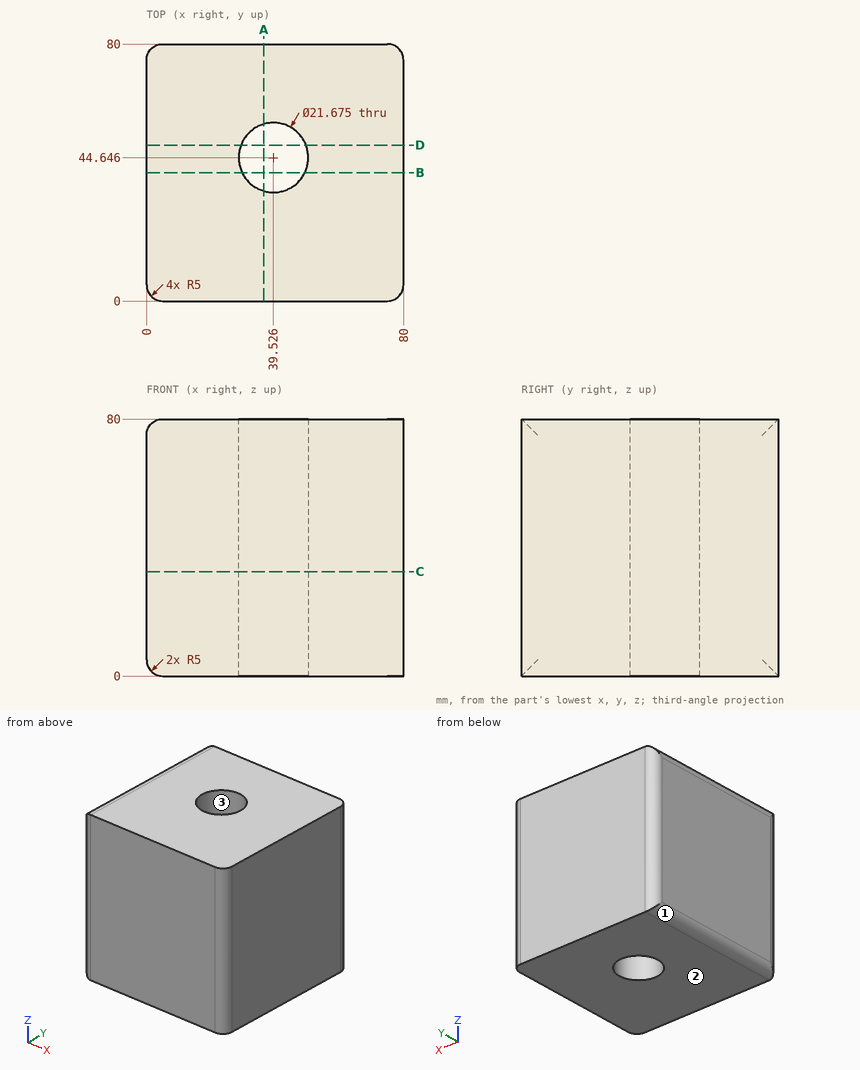
Geometry check sheet. Reference: drawing and pictorial views, mm from the part's lowest x, y, z. Give positions to 0.01 mm unless a question says otherwise; leave off trailing zeros. Loops run counter-clockwise (first coordinate to the right, second up) from the corner with the lowest first, then second, coordinate; pieces in that order, holes last. Notation, with made-up numbers: (26.5, 12.5) - (36.5, 12.5) arc R18 ccw to (36.5, 31.5) - close; hole circle Ø7 at (48, 13). An arc over 180 degrees is marked (long way). Use CSV: the item, a comma, the result in double quotes. Start each with the question number.
Q1. Section check B-B, the plane y = 40. Record the cut outline in (x, z) (1 decimal).
Q2. Section check C-C, the plane z = 32.5. Record the cut outline in (x, y) (1 decimal).
Q3. Scan lines: probe 1 along X at (y, z) = (39, 62) (1 decimal); probe 2 along X at (y, z) = (35.5, 23) (1 decimal); probe 3 along Y at (x, z) = (35, 45). Record each from-to range of solid material in increasing order. Write a range as from..to.
Q4. Section check D-D, the plane y = 48.5. Record the cut outline in (x, z) (1 decimal).
Q5. Release check for a two-part mould opening along X. For the marked faces 1, 2 and 3 record: +X half, -X half, draft (parallel to the pull), parting line (faces both ways), or undercut.
Q6. Section check A-A, the plane x = 36.5. Record the cut outline in (y, z), and give its area (4 significant figures).
Findings below:
1,outline,"(0, 5) arc R5 ccw to (5, 0) - (29.7, 0) - (29.7, 80) - (5, 80) arc R5 ccw to (0, 75) - close; (49.3, 0) - (80, 0) - (80, 80) - (49.3, 80) - close"
2,outline,"(0, 5) arc R5 ccw to (5, 0) - (75, 0) arc R5 ccw to (80, 5) - (80, 75) arc R5 ccw to (75, 80) - (5, 80) arc R5 ccw to (0, 75) - close; hole circle Ø21.7 at (39.5, 44.6)"
3,probe 1,"x = 0..30.3, 48.8..80"
3,probe 2,"x = 0..33.7, 45.3..80"
3,probe 3,"y = 0..34.8, 54.49..80"
4,outline,"(0, 5) arc R5 ccw to (5, 0) - (29.4, 0) - (29.4, 80) - (5, 80) arc R5 ccw to (0, 75) - close; (49.7, 0) - (80, 0) - (80, 80) - (49.7, 80) - close"
5,face 1,"-X half"
5,face 2,"draft"
5,face 3,"undercut"
6,outline,"(0, 0) - (34.24, 0) - (34.24, 80) - (0, 80) - close; (55.05, 0) - (80, 0) - (80, 80) - (55.05, 80) - close"
6,area,"4,735 mm^2"
